from build123d import *

# Parameters (mm, degrees)
F0_R     = 4.875
F0_R_2   = 2.125
F1_DEPTH = 5
F2_R     = 4.875
F3_DEPTH = 25


with BuildPart() as f1:
    # F0 (on Top) → F1 (new body)
    with BuildSketch(Plane.XY):
        with BuildLine():
            Line((-12.5, 27.5), (-12.5, 0))
            Line((-12.5, 0), (-12.5, -7.5))
            ThreePointArc((-12.5, -7.5), (-11.035534, -11.035534), (-7.5, -12.5))
            Line((-7.5, -12.5), (27.5, -12.5))
            Line((27.5, -12.5), (27.5, 7.5))
            Line((27.5, 7.5), (7.5, 7.5))
            Line((7.5, 7.5), (7.5, 27.5))
            Line((7.5, 27.5), (-12.5, 27.5))
        make_face()
        Circle(F0_R, mode=Mode.SUBTRACT)
        with Locations((17.5, 0)):
            Circle(F0_R_2, mode=Mode.SUBTRACT)
        with Locations((0, 17.5)):
            Circle(F0_R_2, mode=Mode.SUBTRACT)
    extrude(amount=F1_DEPTH)

    # F2 (on face) → F3 (join)
    with BuildSketch(Plane(origin=(0, 0, 0), x_dir=(1, 0, 0), z_dir=(0, 0, -1))):
        Polygon((10, -4.142136), (10, 4.142136), (4.142136, 10), (-4.142136, 10), (-10, 4.142136), (-10, -4.142136), (-4.142136, -10), (4.142136, -10), align=None)
        Circle(F2_R, mode=Mode.SUBTRACT)
    extrude(amount=F3_DEPTH)


solid = f1.part
Build history of the part. All positions in model axes, mm. A direction names the side the tool comes from. Round coordinates to 2 decimals unless told otherwise and drop trailing zeros. Write each loop counter-clockwise with the first axis right and the second up, starting at its lowest first coordinate (ties: lowest second). Pieces come first, ordered by that corner, then holes. Notation, with made-up numbers: (12, 33.5) -> (52, 33.5) arc R30 cw to (52, 64.5) -> close; hole circle Ø1 at (7, 18). An arc over 180 degrees is marked (long way). Write item = value, one per line.
(1) Two-plate mould, pull along Y, no slides. Class faces 1 (the face through (27.5, -3, 2)), 2 (the face through (7.03, 7.11, -12.32)), 3 (the face through (0, -10, -12)), 4 (the face through (15.377, 0.093, 2.465)): pulls with the +Y half, pulls with the -Y half, needs draft (parallel to the pull), parting line crosses it, or undercut.
Answer:
face_1 = needs draft
face_2 = pulls with the +Y half
face_3 = pulls with the -Y half
face_4 = undercut
(2) Band-saw the part on C-C (z = -19). Give the cut face in (x, y) (3 decimals), then the cut area to 3 significant figures.
Answer:
outline = (-10, -4.142) -> (-4.142, -10) -> (4.142, -10) -> (10, -4.142) -> (10, 4.142) -> (4.142, 10) -> (-4.142, 10) -> (-10, 4.142) -> close; hole circle Ø9.75 at (0, 0)
area = 257 mm2
(3) Tool access for faces 5 (the face through (-10, 0, -12)), 6 (the face through (18, 7.5, 2)), 7 (the face through (0, 10, -12)), 8 (the face through (7.11, -7.03, -12.32)): list every direction of +Z, -Z, +X, -X, +Y, -Y with a clear straight run to the whole face (end or side of a thin tool).
Answer:
face_5 = -Z, -X, +Y, -Y
face_6 = +Z, -Z, +X, +Y
face_7 = -Z, +X, -X, +Y
face_8 = -Z, +X, -Y
(4) Flat gauge pins, fed straight in: pin 1 (2.5 mm diameter, centred on y = -0.5, z = -11.5, fed in from +X); pin 2 (7 mm diameter, centred on x = 17.5, y = 0, fed in from -Z); pin 3 (1 mm diameter, centred on x = 8.5, z = -7.5, fed in from +Y). Where does each tip first touch, or does it go through?
Answer:
pin_1 = 10
pin_2 = 0
pin_3 = 6.14
(5) Probe L1, parallel to Y at x = 0, z = -13.5 (3 decimals); L2, parallel to Y at x = 0, z = 3.7 (3 decimals). List the from-to ranges inside material, lowest first.
Answer:
L1 = -10 to -4.875, 4.875 to 10
L2 = -12.5 to -4.875, 4.875 to 15.375, 19.625 to 27.5
(6) Band-saw the part on D-D (z = 2.75). Give the cut face in (x, y) (3 decimals).
Answer:
outline = (-12.5, -7.5) arc R5 ccw to (-7.5, -12.5) -> (27.5, -12.5) -> (27.5, 7.5) -> (7.5, 7.5) -> (7.5, 27.5) -> (-12.5, 27.5) -> close; hole circle Ø9.75 at (0, 0); hole circle Ø4.25 at (0, 17.5); hole circle Ø4.25 at (17.5, 0)
(7) Band-saw the part on A-A (y = 17.5). Give the cut face in (x, z) (3 decimals), then the cut area to 4 significant figures.
Answer:
outline = (-12.5, 0) -> (-2.125, 0) -> (-2.125, 5) -> (-12.5, 5) -> close; (2.125, 0) -> (7.5, 0) -> (7.5, 5) -> (2.125, 5) -> close
area = 78.75 mm2
(8) Band-saw the part on B-B (x = 0). Give the cut face in (y, z) (3 decimals).
Answer:
outline = (-12.5, 0) -> (-10, 0) -> (-10, -25) -> (-4.875, -25) -> (-4.875, 5) -> (-12.5, 5) -> close; (4.875, -25) -> (10, -25) -> (10, 0) -> (15.375, 0) -> (15.375, 5) -> (4.875, 5) -> close; (19.625, 0) -> (27.5, 0) -> (27.5, 5) -> (19.625, 5) -> close
